Design review of the part built by this model. Coordinates are the model's own, in mm. Face numbers are marked on the shaded views. A direction names the side the tool comes from. Coordinates: 2 decimals unless noted, no trailing zeros. Write each loop counter-clockwise with the first axis right and the second up, starting at its lowest first coordinate (ties: lowest second). Pieces come first, ordered by that corner, then holes.
Q1. Add section A-A, the plane y = 4.45. Give the boundary of the cut face in (x, z), plus the area to 3 significant figures.
Q2. Add section C-C, the plane x = -7. Give the boundary of the cut face in (y, z).
Q3. Add section B-B, the plane x = -4.5. Give the boundary of the cut face in (y, z).
Q4. To check wall thickness, follow probe 1 along Z at (x, y) = (0.5, 2.1); probe 2 along Z at (x, y) = (9.75, 3.8); probe 3 along Z at (x, y) = (-11.5, 0.35). State the ranges of each line that lie inside material, in increasing order.
Q5. Machinability: for the marked faces 5, 6 and 7, which of the approach directions +Z, -Z, +X, -X, +Y, -Y give a long, thin tool a straight path to every point of the face, cutting with its end or side? Answer none if there is none.
Q6. Clearance check with flat-ended pins moving along their axes: pin 1 Ø2 at (y, z) = (1.5, -3.5) entering from +X; pin 2 Ø1 at (x, y) = (6.5, 1.5) entering from -Z; pin 3 Ø3 at (x, y) = (2, 1.5) entering from -Z. State where each tip first meets the part, or that it passes through.
Q7. The part is to be moulded in two halves that separate along Z. For the marked faces 1, 2, 3 and 4, say which applies: +Z half, -Z half, draft (parallel to the pull), parting line (faces both ways), or undercut.
Autodesk Inventor part; units mm, degrees
ref_plane "YZ Plane" through (0, 0, 0) normal (1, 0, 0) x (0, 1, 0)
ref_plane "XZ Plane" through (0, 0, 0) normal (0, 1, 0) x (-1, 0, 0)
ref_plane "XY Plane" through (0, 0, 0) normal (0, 0, 1) x (1, 0, 0)
sketch "Sketch1" plane through (0, 0, 0) normal (0, 1, 0) x (-1, 0, 0)
  circle A0 centre (0, 0) radius 8.5
  line L0 (7.953, 3) -> (12.5, 1.5)
  line L1 (12.5, 1.5) -> (12.5, -1.5)
  line L2 (12.5, -1.5) -> (7.953, -3)
  line L3 (5.2893, 11.4247) -> (5.3108, 6.6367)
  line L4 (-0.3956, 8.4908) -> (2.4361, 12.3517)
  line L5 (2.4361, 12.3517) -> (5.2893, 11.4247)
  line L6 (-9.231, 8.5608) -> (-4.6707, 7.1017)
  line L7 (-8.1975, 2.2476) -> (-10.9944, 6.1338)
  line L8 (-10.9944, 6.1338) -> (-9.231, 8.5608)
  line L9 (-10.9944, -6.1338) -> (-8.1975, -2.2476)
  line L10 (-4.6707, -7.1017) -> (-9.231, -8.5608)
  line L11 (-9.231, -8.5608) -> (-10.9944, -6.1338)
  line L12 (2.4361, -12.3517) -> (-0.3956, -8.4908)
  line L13 (5.3108, -6.6367) -> (5.2893, -11.4247)
  line L14 (5.2893, -11.4247) -> (2.4361, -12.3517)
  point P0 (-0.3956, -8.4908)
  dimension "d0" = 17
  dimension "d1" = 3
  dimension "d2" = 4
  dimension "d3" = 6
  dimension "d4" = 108.257
  dimension "d5" = 108.257
  dimension "d8" = 360
extrude "Extrusion1" add sketch "Sketch1" along normal blind 5
equation "\"d4\" = d5"
properties part number "AP-1-01-spur5tooth"
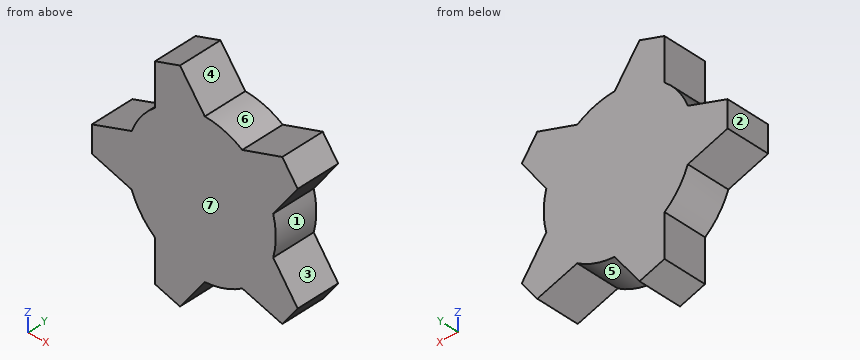
Here are the results:
1. outline: (-12.5, -1.5) - (-7.95, -3) arc R8.5 ccw to (-5.31, -6.64) - (-5.29, -11.42) - (-2.44, -12.35) - (0.4, -8.49) arc R8.5 ccw to (4.67, -7.1) - (9.23, -8.56) - (10.99, -6.13) - (8.2, -2.25) arc R8.5 ccw to (8.2, 2.25) - (10.99, 6.13) - (9.23, 8.56) - (4.67, 7.1) arc R8.5 ccw to (0.4, 8.49) - (-2.44, 12.35) - (-5.29, 11.42) - (-5.31, 6.64) arc R8.5 ccw to (-7.95, 3) - (-12.5, 1.5) - close
1. area: 318 mm2
2. outline: (0, -4.82) - (5, -4.82) - (5, 4.82) - (0, 4.82) - close
3. outline: (0, -11.68) - (5, -11.68) - (5, 11.68) - (0, 11.68) - close
4. probe 1: z = -8.49 to 8.49
4. probe 2: z = -7.85 to -4.4, 4.4 to 7.85
4. probe 3: z = -1.83 to 1.83
5. face 5: -Z, +Y, -Y
5. face 6: +Z, +Y, -Y
5. face 7: +Z, -Z, +X, -X, -Y
6. pin 1: stops at x = 9.82
6. pin 2: stops at z = -7.85
6. pin 3: stops at z = -8.49
7. face 1: undercut
7. face 2: draft
7. face 3: undercut
7. face 4: +Z half
